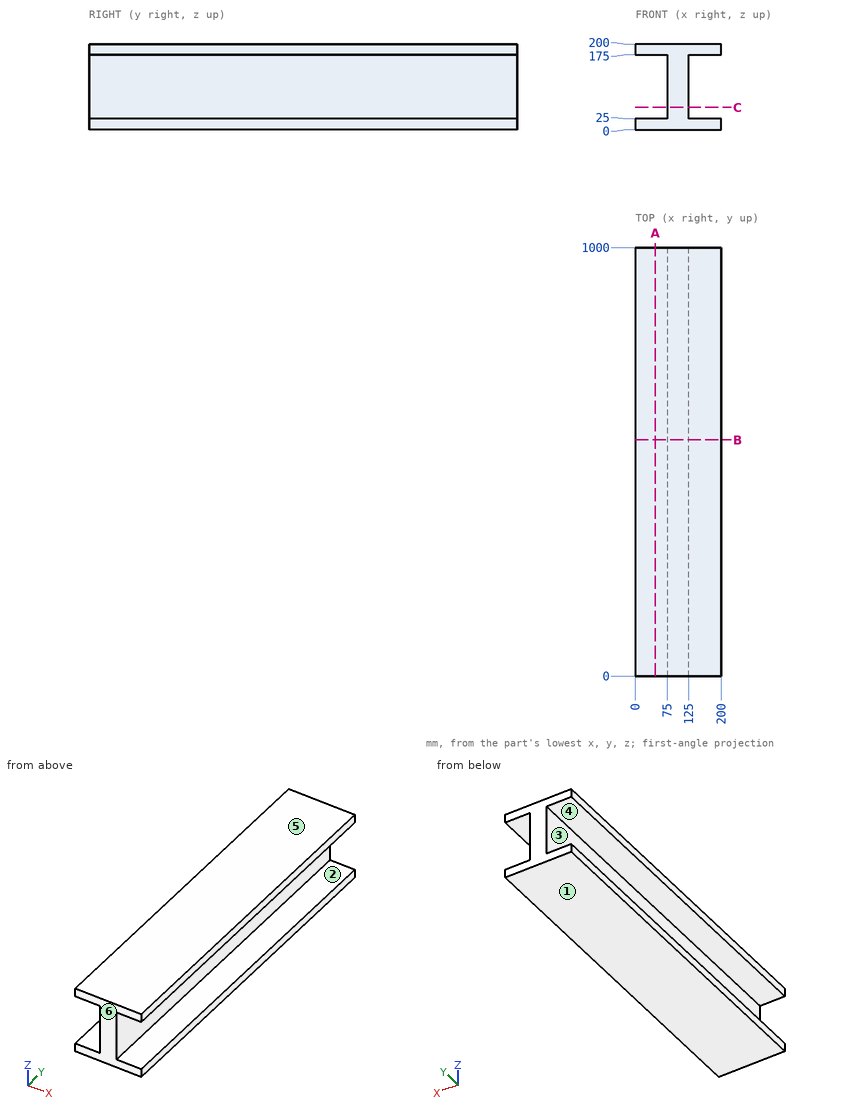
For this review, use the dimensioned drawing (mm, ordinates from the lowest corner) and the shaded views. A direction names the side the tool comes from. Round coordinates to 2 decimals unless told otherwise and drop trailing zeros. Order: outer loops, then holes, each group sorted by start corner. A loop starts at its lowest first (then second) coordinate and runs counter-clockwise, first axis right, second up.
1) Consider section B-B (y = 551.5). State the section outline as (x, z) points.
The answers:
outline: (0, 0) - (200, 0) - (200, 25) - (125, 25) - (125, 175) - (200, 175) - (200, 200) - (0, 200) - (0, 175) - (75, 175) - (75, 25) - (0, 25) - close
2) Consider section C-C (z = 52). State the section outline as (x, y) points, plus the area to 3 significant figures.
The answers:
outline: (75, 0) - (125, 0) - (125, 1000) - (75, 1000) - close
area: 50,000 mm2
3) Machinability: for the marked faces 1, 2 and 3, which of the approach directions +Z, -Z, +X, -X, +Y, -Y give a long, thin tool a straight path to every point of the face, cutting with its end or side? Answer none if there is none.
The answers:
face 1: -Z, +X, -X, +Y, -Y
face 2: +X, +Y, -Y
face 3: -X, +Y, -Y
4) For L1, parallel to Z at x = 48, y = 448; L2, parallel to X at y = 217.5, z = 75.5, list the stretches that pass through material, from the lowest coordinate up.
The answers:
L1: z = 0 to 25, 175 to 200
L2: x = 75 to 125
5) Clearance check with a flat-ended pin moving along its axis: pin 1 Ø1.5 at (y, z) = (793.5, 67.5) entering from +X. State where the tip first meets the part, or that it passes through.
The answers:
pin 1: stops at x = 125
6) Draft analysis for pull direction Z (two halves, no side actions). For the marked faces 4, 5 and 6, state which applies: released by +Z, released by -Z, zero draft, split by the parting line, or undercut.
The answers:
face 4: undercut
face 5: released by +Z
face 6: zero draft
7) Consider section A-A (x = 47). State the section outline as (y, z) points, plus the area to 3 significant figures.
The answers:
outline: (0, 0) - (1000, 0) - (1000, 25) - (0, 25) - close; (0, 175) - (1000, 175) - (1000, 200) - (0, 200) - close
area: 50,000 mm2
